The model under review builds one solid part; all positions refer to its coordinate system, in mm. A direction names the side the tool comes from. Give positions to 0.01 mm unless a question says otherwise; leave off trailing zeros. Write each loop counter-clockwise with the first axis right and the second up, starting at its lowest first coordinate (ties: lowest second). Pieces come first, ordered by that corner, then holes. Notation, with made-up numbers: (-17.75, -22.75) -> (22.25, -22.75) arc R18 cw to (22.25, 7.25) -> close; hole circle Ø7 at (63.5, 45.5). An arc over 180 degrees is marked (long way). Use CSV: the item, a comma, the result in double quotes.
```python
from build123d import *

# Parameters (mm, degrees)
CROQUIS1_R              = 11.5
SALIENTE_EXTRUIR1_DEPTH = 2
CROQUIS1_9_R            = 0.75
CORTAR_EXTRUIR2_DEPTH   = 3
MATRIZC2_COUNT          = 4
SALIENTE_EXTRUIR2_START = 2
CROQUIS1_11_R           = 5
SALIENTE_EXTRUIR2_DEPTH = 1.5
SALIENTE_EXTRUIR3_START = 3.5
CROQUIS1_12_R           = 2
SALIENTE_EXTRUIR3_DEPTH = 3
REDONDEO1_R             = 0.5
CROQUIS1_13_R           = 5
CROQUIS1_13_R_2         = 2
SALIENTE_EXTRUIR4_DEPTH = 1


with BuildPart() as part:
    # Croquis1 → Saliente-Extruir1 (new body)
    with BuildSketch(Plane(origin=(0, 0, 0), x_dir=(1, 0, 0), z_dir=(0, 1, 0))):
        with Locations((0, 13.3)):
            Circle(CROQUIS1_R)
    extrude(amount=SALIENTE_EXTRUIR1_DEPTH)

    # Croquis1<9> → Cortar-Extruir2 (cut)
    with BuildSketch(Plane(origin=(0, 0, 0), x_dir=(1, 0, 0), z_dir=(0, 1, 0))):
        with Locations((0, 22.3)):
            Circle(CROQUIS1_9_R)
        with Locations((3, 21.785281374)):
            Circle(CROQUIS1_9_R)
        with Locations((-3, 21.785281374)):
            Circle(CROQUIS1_9_R)
    cortar_extruir2 = extrude(amount=CORTAR_EXTRUIR2_DEPTH, mode=Mode.SUBTRACT)

    # MatrizC2: Cortar-Extruir2 ×4 about axis
    matrizc2_axis = Axis((0, 0, -13.3), (0, 1, 0))
    for i in range(1, MATRIZC2_COUNT):
        add(cortar_extruir2.rotate(matrizc2_axis, i * 360 / MATRIZC2_COUNT), mode=Mode.SUBTRACT)

    # Croquis1<11> → Saliente-Extruir2 (add)
    with BuildSketch(Plane(origin=(0, 0, 0), x_dir=(1, 0, 0), z_dir=(0, 1, 0)).offset(SALIENTE_EXTRUIR2_START)):
        with Locations((0, 13.3)):
            Circle(CROQUIS1_11_R)
    extrude(amount=SALIENTE_EXTRUIR2_DEPTH)

    # Croquis1<12> → Saliente-Extruir3 (add)
    with BuildSketch(Plane(origin=(0, 0, 0), x_dir=(1, 0, 0), z_dir=(0, 1, 0)).offset(SALIENTE_EXTRUIR3_START)):
        with Locations((0, 13.3)):
            Circle(CROQUIS1_12_R)
        Polygon((1, 12.722649731), (1, 13.877350269), (0, 14.454700538), (-1, 13.877350269), (-1, 12.722649731), (0, 12.145299462), align=None, mode=Mode.SUBTRACT)
    extrude(amount=SALIENTE_EXTRUIR3_DEPTH)

    # Redondeo1
    redondeo1_edges = [part.edges().sort_by_distance(p)[0] for p in [
        (-11.5, 2, -13.3),
        (-5, 3.5, -13.3),
        (-2, 6.5, -13.3),
    ]]
    fillet(redondeo1_edges, radius=REDONDEO1_R)

    # Croquis1<13> → Saliente-Extruir4 (add)
    with BuildSketch(Plane(origin=(0, 0, 0), x_dir=(1, 0, 0), z_dir=(0, 1, 0))):
        with Locations((0, 13.3)):
            Circle(CROQUIS1_13_R)
        with Locations((0, 13.3)):
            Circle(CROQUIS1_13_R_2, mode=Mode.SUBTRACT)
    extrude(amount=-SALIENTE_EXTRUIR4_DEPTH)


solid = part.part
```
Q1. The part is to be moulded in two halves that separate along X. For faces 4 (the flat face through (2, 3.5, -12)), 5 (the cylindrical face through (-4, -0.5, -10.3)), 6 (the flat face through (1, 5, -13)), say which applies: pulls with the +X half, pulls with the -X half, needs draft (parallel to the pull), parting line crosses it, or undercut.
Derived:
face 4,"needs draft"
face 5,"parting line crosses it"
face 6,"undercut"
Q2. Consider section B-B (y = 0.5). State how many separate pieces and enclosed holes the cut face has, then the cut area to 3 significant figures.
Derived:
separate pieces,"1"
enclosed holes,"12"
area,"394 mm2"
Q3. To check wall thickness, follow probe 1 along Z at (x, y) = (0, 1.45); probe 2 along Z at (x, y) = (9, 1.1); probe 3 along X at (y, z) = (1.1, -16.3). State the ranges of each line that lie inside material, in increasing order.
Derived:
probe 1,"z = -24.8 to -23.05, -21.55 to -5.05, -3.55 to -1.8"
probe 2,"z = -20.46 to -16.85, -15.75 to -14.05, -12.55 to -10.85, -9.75 to -6.14"
probe 3,"x = -11.1 to -9.24, -7.74 to 7.74, 9.24 to 11.1"
Q4. Machinability: for faces 1 (the cylindrical face through (-3.595, 0.986, -21.329)), 2 (the flat face through (5, 0, -11)), 3 (the flat face through (0.51, 4.98, -14.16)), which of the approach directions +Z, -Z, +X, -X, +Y, -Y give a long, thin tool a straight path to every point of the face, cutting with its end or side? Answer none if there is none.
Derived:
face 1,"+Y, -Y"
face 2,"-Y"
face 3,"+Y"
Q5. Consider section A-A (y = 4). Write out the cut boundary in (x, z), then the cut area to 3 significant figures.
Derived:
outline,"circle Ø4 at (0, -13.3); hole (-1, -13.88) -> (0, -14.45) -> (1, -13.88) -> (1, -12.72) -> (0, -12.15) -> (-1, -12.72) -> close"
area,"9.10 mm2"
Q6. Insertion check: pin 1 (1.4 mm diameter, centred on x = 8.49, z = -10.3, fed in from -Y); pin 2 (4.5 mm diameter, centred on x = -0.5, z = -13.5, fed in from +Y); pin 3 (3 mm diameter, centred on x = -3.5, z = -6, fed in from -Y); pin 4 (3 mm diameter, centred on y = 4.5, z = -18, fed in from +X). Each pin has a flat end and moves straight along its axis. Give the tip position at first contact, or say it passes through.
Derived:
pin 1,"passes through"
pin 2,"stops at y = 6.5"
pin 3,"stops at y = 0"
pin 4,"stops at x = 3.1"
